```python
from build123d import *

# Parameters (mm, degrees)
F0_W     = 106.410607
F0_H     = 65.193332
F1_DEPTH = 25.4
F2_R     = 14.819115
F3_DEPTH = 125.476


with BuildPart() as f1:
    # F0 (on Top) → F1 (new body)
    with BuildSketch(Plane.XY):
        with Locations((-8.485909, 0)):
            Rectangle(F0_W, F0_H)
    extrude(amount=F1_DEPTH)

    # F2 (on face) → F3 (cut)
    with BuildSketch(Plane.XY.offset(25.4)):
        Circle(F2_R)
    extrude(amount=-F3_DEPTH, mode=Mode.SUBTRACT)


solid = f1.part
```
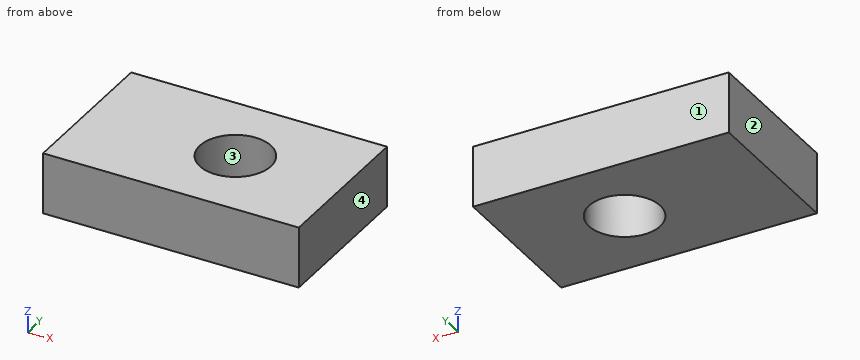
Read the model definition and answer for the solid it produces. Units are mm, in the model's axes. Face numbers are marked on the shaded views. Give positions to 0.01 mm unless a question says otherwise; leave off trailing zeros. Order: outer loops, then holes, each group sorted by start corner. A loop starts at its lowest first (then second) coordinate and runs counter-clockwise, first axis right, second up.
(1) Given pin 1 (18 mm diameter, centred on x = 0, y = 0, fed in from -Z), flat-ended and moving along its own axis, determine where the tip first touches the part or whether it passes through.
(2) Find section A-A (y = 0). Give the vertices of the cut face in (x, z), plus the area to 3 significant figures.
(3) For a pull along X with two mould halves and no side action, classify the marked faces 1, 2, 3 and 4 as released by +X, released by -X, zero draft, split by the parting line, or undercut.
(4) Straight lines are drawn through the part: L1, parallel to Y at x = 0, z = 19.25; L2, parallel to X at y = 3, z = 19.25; L3, parallel to X at y = -11.5, z = 17.75. For each, find the intervals that lie inside material, in ascending order.
(5) Find section B-B (x = -13). Give the vertices of the cut face in (y, z).
(6) Find section C-C (z = 6.5). Give the vertices of the cut face in (x, y), plus the area to 3 significant figures.
Result sheet:
1. pin 1: passes through
2. outline: (-61.69, 0) - (-14.82, 0) - (-14.82, 25.4) - (-61.69, 25.4) - close; (14.82, 0) - (44.72, 0) - (44.72, 25.4) - (14.82, 25.4) - close
2. area: 1,950 mm2
3. face 1: zero draft
3. face 2: released by -X
3. face 3: undercut
3. face 4: released by +X
4. L1: y = -32.6 to -14.82, 14.82 to 32.6
4. L2: x = -61.69 to -14.51, 14.51 to 44.72
4. L3: x = -61.69 to -9.35, 9.35 to 44.72
5. outline: (-32.6, 0) - (-7.11, 0) - (-7.11, 25.4) - (-32.6, 25.4) - close; (7.11, 0) - (32.6, 0) - (32.6, 25.4) - (7.11, 25.4) - close
6. outline: (-61.69, -32.6) - (44.72, -32.6) - (44.72, 32.6) - (-61.69, 32.6) - close; hole circle Ø29.64 at (0, 0)
6. area: 6,250 mm2
